from build123d import *

# Parameters (mm, degrees)
SKETCH_W      = 32
SKETCH_H      = 80
PAD_DEPTH     = 12
SKETCH001_R   = 2.55
HOLE_DEPTH    = 25
SKETCH002_R   = 3
HOLE001_DEPTH = 12.001
SKETCH003_R   = 3
HOLE002_DEPTH = 25
FILLET_R      = 2
FILLET001_R   = 1
POCKET_DEPTH  = 6


with BuildPart() as part:
    # Sketch → Pad (new body)
    with BuildSketch(Plane.XZ):
        Rectangle(SKETCH_W, SKETCH_H)
    extrude(amount=-PAD_DEPTH)

    # Sketch001 → Hole (cut)
    with BuildSketch(Plane.XZ):
        with Locations((0, 30)):
            Circle(SKETCH001_R)
        with Locations((0, -30)):
            Circle(SKETCH001_R)
    extrude(amount=-HOLE_DEPTH, mode=Mode.SUBTRACT)

    # Sketch002 → Hole001 (cut, through all)
    with BuildSketch(Plane.XZ):
        with Locations((0, 20)):
            Circle(SKETCH002_R)
        with Locations((0, -20)):
            Circle(SKETCH002_R)
    extrude(amount=-HOLE001_DEPTH, mode=Mode.SUBTRACT)

    # Sketch003 → Hole002 (cut)
    with BuildSketch(Plane.XZ):
        Circle(SKETCH003_R)
    extrude(amount=-HOLE002_DEPTH, mode=Mode.SUBTRACT)

    # Fillet
    fillet_edges = [part.edges().sort_by_distance(p)[0] for p in [
        (-16, 6, 40),
        (16, 6, 40),
        (16, 6, -40),
        (-16, 6, -40),
    ]]
    fillet(fillet_edges, radius=FILLET_R)

    # Fillet001
    fillet001_edges = [part.edges().sort_by_distance(p)[0] for p in [
        (0, 0, -40),
        (-15.414214, 0, -39.414214),
        (-16, 0, 0),
        (-15.414214, 0, 39.414214),
        (0, 0, 40),
        (15.414214, 0, 39.414214),
        (16, 0, 0),
        (15.414214, 0, -39.414214),
    ]]
    fillet(fillet001_edges, radius=FILLET001_R)

    # Sketch004 → Pocket (cut)
    with BuildSketch(Plane.XZ):
        Polygon((2.944486, 25.1), (-2.944486, 25.1), (-5.888973, 20), (-2.944486, 14.9), (2.944486, 14.9), (5.888973, 20), align=None)
        Polygon((2.944486, -14.9), (-2.944486, -14.9), (-5.888973, -20), (-2.944486, -25.1), (2.944486, -25.1), (5.888973, -20), align=None)
    extrude(amount=-POCKET_DEPTH, mode=Mode.SUBTRACT)


solid = part.part
Read the model definition and answer for the solid it produces. Units are mm, in the model's axes. A direction names the side the tool comes from. Round coordinates to 2 decimals unless told otherwise and drop trailing zeros. Order: outer loops, then holes, each group sorted by start corner. A loop starts at its lowest first (then second) coordinate and runs counter-clockwise, first axis right, second up. Notation, with made-up numbers: (-27, 74.5) - (1, 74.5) arc R18 ccw to (1, 107.5) - close; hole circle Ø11 at (25, 55.25). An arc over 180 degrees is marked (long way). Use one line per item in the form item = value. Start each with the question number.
(1) A flat-ended cylindrical pin translates along its axis: pin 1 Ø3 at (x, z) = (0, -18) entering from -Y. Find the tip coordinate at first contact, or state that the pin passes through.
(2) The part is cut by section B-B (z = -30). Give the vertices of the cut face in (x, y).
(3) The part is cut by section C-C (y = 11). Give the vertices of the cut face in (x, z), then the cut area to 3 significant figures.
(4) Find the intervals of material crossed by line 1 along Z through (x, y) = (0, 8.9); line 2 along Z through (x, y) = (0, 4.25); line 3 along X through (y, z) = (5.5, -31.5), in increasing order. Write a range as from..to.
(5) For faces 5 (the face through (3, 6, 22)), 6 (the face through (-16, 6, -1)), determine the directions among +Z, -Z, +X, -X, +Y, -Y from which every point of the face is accessible in a straight line to the end or side of a thin tool.
(6) Determine the mould class of faces 1 (the face through (0, 3, 14.9)), 2 (the face through (16, 6, -1)), 3 (the face through (15.4, 6.58, 39.43)), 4 (the face through (0, 6, -40)) for opening direction Z: +Z half, -Z half, draft (parallel to the pull), parting line (faces both ways), or undercut.
(7) The part is cut by section A-A (y = 3.25). Give the vertices of the cut face in (x, z).
Checked values:
q1.pin_1 = 6
q2.outline = (-16, 1) arc R1 ccw to (-15, 0) - (-2.55, 0) - (-2.55, 12) - (-16, 12) - close; (2.55, 0) - (15, 0) arc R1 ccw to (16, 1) - (16, 12) - (2.55, 12) - close
q3.outline = (-16, -38) arc R2 ccw to (-14, -40) - (14, -40) arc R2 ccw to (16, -38) - (16, 38) arc R2 ccw to (14, 40) - (-14, 40) arc R2 ccw to (-16, 38) - close; hole circle Ø6 at (0, -20); hole circle Ø6 at (0, 0); hole circle Ø6 at (0, 20); hole circle Ø5.1 at (0, -30); hole circle Ø5.1 at (0, 30)
q3.area = 2,430 mm^2
q4.line_1 = -40..-32.55, -27.45..-23, -17..-3, 3..17, 23..27.45, 32.55..40
q4.line_2 = -40..-32.55, -27.45..-25.1, -14.9..-3, 3..14.9, 25.1..27.45, 32.55..40
q4.line_3 = -16..-2.06, 2.06..16
q5.face_5 = -Y
q5.face_6 = +Z, -Z, -X, +Y, -Y
q6.face_1 = undercut
q6.face_2 = draft
q6.face_3 = +Z half
q6.face_4 = -Z half
q7.outline = (-16, -38) arc R2 ccw to (-14, -40) - (14, -40) arc R2 ccw to (16, -38) - (16, 38) arc R2 ccw to (14, 40) - (-14, 40) arc R2 ccw to (-16, 38) - close; hole (-5.89, -20) - (-2.94, -25.1) - (2.94, -25.1) - (5.89, -20) - (2.94, -14.9) - (-2.94, -14.9) - close; hole (-5.89, 20) - (-2.94, 14.9) - (2.94, 14.9) - (5.89, 20) - (2.94, 25.1) - (-2.94, 25.1) - close; hole circle Ø6 at (0, 0); hole circle Ø5.1 at (0, -30); hole circle Ø5.1 at (0, 30)
